Can you work these out from the model? Positions are in its coordinate system, mm. Face numbers are marked on the shaded views. A direction names the side the tool comes from. Give positions to 0.01 mm unless a question says otherwise; leave off trailing zeros. Loops run counter-clockwise (first coordinate to the right, second up) from the corner with the lowest first, then second, coordinate; pieces in that order, holes last. Notation, with made-up numbers: (68.25, 10.5) -> (84.25, 10.5) arc R27 cw to (84.25, 34.5) -> close; hole circle Ø8 at (7, 52.25). An arc over 180 degrees is marked (long way). Use CSV: the item, a comma, the result in double quotes.
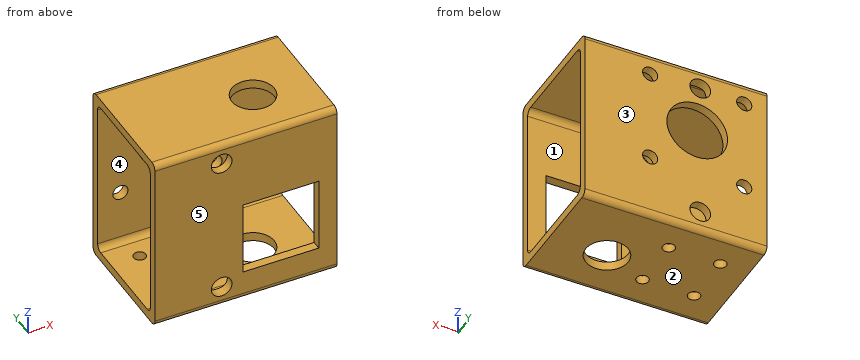
from build123d import *

# Parameters (mm, degrees)
EXTRUDE_1_DEPTH     = 60
CUT_EXTRUDE_1_REACH = 42
SKETCH_2_R          = 2.5
SKETCH_2_R_2        = 10
SKETCH_3_R          = 7
CUT_EXTRUDE_2_DEPTH = 61
HOLE_WIZARD_M8_1_D  = 6.8
CUT_EXTRUDE_3_REACH = 62
SKETCH_6_R          = 2
CUT_EXTRUDE_4_REACH = 42
SKETCH_7_W          = 25
SKETCH_7_H          = 25


with BuildPart() as part:
    # 草图1 → 凸台-拉伸1 (new body)
    with BuildSketch(Plane(origin=(0, 0, 0), x_dir=(0, 0, -1), z_dir=(1, 0, 0))):
        with BuildLine():
            Line((60, 2), (60, 38))
            ThreePointArc((60, 38), (59.414213562, 39.414213562), (58, 40))
            Line((58, 40), (2, 40))
            ThreePointArc((2, 40), (0.585786438, 39.414213562), (0, 38))
            Line((0, 38), (0, 2))
            ThreePointArc((0, 2), (0.585786438, 0.585786438), (2, 0))
            Line((2, 0), (58, 0))
            ThreePointArc((58, 0), (59.414213562, 0.585786438), (60, 2))
        make_face()
        with BuildLine():
            Line((3, 5), (3, 35))
            ThreePointArc((3, 35), (3.585786438, 36.414213562), (5, 37))
            Line((5, 37), (55, 37))
            ThreePointArc((55, 37), (56.414213562, 36.414213562), (57, 35))
            Line((57, 35), (57, 5))
            ThreePointArc((57, 5), (56.414213562, 3.585786438), (55, 3))
            Line((55, 3), (5, 3))
            ThreePointArc((5, 3), (3.585786438, 3.585786438), (3, 5))
        make_face(mode=Mode.SUBTRACT)
    extrude(amount=EXTRUDE_1_DEPTH)

    # 草图2 → 切除-拉伸1 (cut, up to next)
    with BuildSketch(Plane(origin=(0, 40, 0), x_dir=(1, 0, 0), z_dir=(0, 1, 0)), mode=Mode.PRIVATE) as cut_extrude_1_sk1:
        with Locations((7.5, 7.5)):
            Circle(SKETCH_2_R)
    cut_extrude_1_tool1 = extrude(cut_extrude_1_sk1.sketch, amount=-CUT_EXTRUDE_1_REACH, mode=Mode.PRIVATE) & part.part
    add(cut_extrude_1_tool1.solids().sort_by_distance((7.5, 40, -7.5))[0], mode=Mode.SUBTRACT)
    # 草图2 → 切除-拉伸1 (cut, up to next)
    with BuildSketch(Plane(origin=(0, 40, 0), x_dir=(1, 0, 0), z_dir=(0, 1, 0)), mode=Mode.PRIVATE) as cut_extrude_1_sk2:
        with Locations((38.5, 7.5)):
            Circle(SKETCH_2_R)
    cut_extrude_1_tool2 = extrude(cut_extrude_1_sk2.sketch, amount=-CUT_EXTRUDE_1_REACH, mode=Mode.PRIVATE) & part.part
    add(cut_extrude_1_tool2.solids().sort_by_distance((38.5, 40, -7.5))[0], mode=Mode.SUBTRACT)
    # 草图2 → 切除-拉伸1 (cut, up to next)
    with BuildSketch(Plane(origin=(0, 40, 0), x_dir=(1, 0, 0), z_dir=(0, 1, 0)), mode=Mode.PRIVATE) as cut_extrude_1_sk3:
        with Locations((38.5, 38.5)):
            Circle(SKETCH_2_R)
    cut_extrude_1_tool3 = extrude(cut_extrude_1_sk3.sketch, amount=-CUT_EXTRUDE_1_REACH, mode=Mode.PRIVATE) & part.part
    add(cut_extrude_1_tool3.solids().sort_by_distance((38.5, 40, -38.5))[0], mode=Mode.SUBTRACT)
    # 草图2 → 切除-拉伸1 (cut, up to next)
    with BuildSketch(Plane(origin=(0, 40, 0), x_dir=(1, 0, 0), z_dir=(0, 1, 0)), mode=Mode.PRIVATE) as cut_extrude_1_sk4:
        with Locations((7.5, 38.5)):
            Circle(SKETCH_2_R)
    cut_extrude_1_tool4 = extrude(cut_extrude_1_sk4.sketch, amount=-CUT_EXTRUDE_1_REACH, mode=Mode.PRIVATE) & part.part
    add(cut_extrude_1_tool4.solids().sort_by_distance((7.5, 40, -38.5))[0], mode=Mode.SUBTRACT)
    # 草图2 → 切除-拉伸1 (cut, up to next)
    with BuildSketch(Plane(origin=(0, 40, 0), x_dir=(1, 0, 0), z_dir=(0, 1, 0)), mode=Mode.PRIVATE) as cut_extrude_1_sk5:
        with Locations((23, 23)):
            Circle(SKETCH_2_R_2)
    cut_extrude_1_tool5 = extrude(cut_extrude_1_sk5.sketch, amount=-CUT_EXTRUDE_1_REACH, mode=Mode.PRIVATE) & part.part
    add(cut_extrude_1_tool5.solids().sort_by_distance((23, 40, -23))[0], mode=Mode.SUBTRACT)

    # 草图3 → 切除-拉伸2 (cut, through all)
    with BuildSketch(Plane.XY):
        with Locations((41, 17)):
            Circle(SKETCH_3_R)
    extrude(amount=-CUT_EXTRUDE_2_DEPTH, mode=Mode.SUBTRACT)

    # M8 螺纹孔1 (through all)
    with Locations(Plane(origin=(0, 40, 0), x_dir=(1, 0, 0), z_dir=(0, 1, 0))):
        with Locations((22, 53), (22, 7)):
            Hole(HOLE_WIZARD_M8_1_D / 2)

    # 草图6 → 切除-拉伸3 (cut, up to next)
    with BuildSketch(Plane(origin=(0, 0, -60), x_dir=(-1, 0, 0), z_dir=(0, 0, -1)), mode=Mode.PRIVATE) as cut_extrude_3_sk1:
        with Locations((-9.514718626, 11.514718626)):
            Circle(SKETCH_6_R)
    cut_extrude_3_tool1 = extrude(cut_extrude_3_sk1.sketch, amount=-CUT_EXTRUDE_3_REACH, mode=Mode.PRIVATE) & part.part
    add(cut_extrude_3_tool1.solids().sort_by_distance((9.514719, 11.514719, -60))[0], mode=Mode.SUBTRACT)
    # 草图6 → 切除-拉伸3 (cut, up to next)
    with BuildSketch(Plane(origin=(0, 0, -60), x_dir=(-1, 0, 0), z_dir=(0, 0, -1)), mode=Mode.PRIVATE) as cut_extrude_3_sk2:
        with Locations((-26.485281374, 11.514718626)):
            Circle(SKETCH_6_R)
    cut_extrude_3_tool2 = extrude(cut_extrude_3_sk2.sketch, amount=-CUT_EXTRUDE_3_REACH, mode=Mode.PRIVATE) & part.part
    add(cut_extrude_3_tool2.solids().sort_by_distance((26.485281, 11.514719, -60))[0], mode=Mode.SUBTRACT)
    # 草图6 → 切除-拉伸3 (cut, up to next)
    with BuildSketch(Plane(origin=(0, 0, -60), x_dir=(-1, 0, 0), z_dir=(0, 0, -1)), mode=Mode.PRIVATE) as cut_extrude_3_sk3:
        with Locations((-26.485281374, 28.485281374)):
            Circle(SKETCH_6_R)
    cut_extrude_3_tool3 = extrude(cut_extrude_3_sk3.sketch, amount=-CUT_EXTRUDE_3_REACH, mode=Mode.PRIVATE) & part.part
    add(cut_extrude_3_tool3.solids().sort_by_distance((26.485281, 28.485281, -60))[0], mode=Mode.SUBTRACT)
    # 草图6 → 切除-拉伸3 (cut, up to next)
    with BuildSketch(Plane(origin=(0, 0, -60), x_dir=(-1, 0, 0), z_dir=(0, 0, -1)), mode=Mode.PRIVATE) as cut_extrude_3_sk4:
        with Locations((-9.514718626, 28.485281374)):
            Circle(SKETCH_6_R)
    cut_extrude_3_tool4 = extrude(cut_extrude_3_sk4.sketch, amount=-CUT_EXTRUDE_3_REACH, mode=Mode.PRIVATE) & part.part
    add(cut_extrude_3_tool4.solids().sort_by_distance((9.514719, 28.485281, -60))[0], mode=Mode.SUBTRACT)

    # 草图7 → 切除-拉伸4 (cut, up to next)
    with BuildSketch(Plane.XZ, mode=Mode.PRIVATE) as cut_extrude_4_sk1:
        with Locations((41.5, -37.5)):
            Rectangle(SKETCH_7_W, SKETCH_7_H)
    cut_extrude_4_tool1 = extrude(cut_extrude_4_sk1.sketch, amount=-CUT_EXTRUDE_4_REACH, mode=Mode.PRIVATE) & part.part
    add(cut_extrude_4_tool1.solids().sort_by_distance((41.5, 0, -37.5))[0], mode=Mode.SUBTRACT)


solid = part.part
(1) Which directions (+Z, -Z, +X, -X, +Y, -Y) give clear straight access to the entire face, cutting with the end or side of a thin tool? Please do the marked faces 4 and 5.
Answer sheet:
face 4,"+X, -X"
face 5,"+Z, -Z, +X, -X, -Y"
(2) Will these pins go through, and if not, where does the flat tip stop? pin 1 Ø4 at (x, z) = (47, -37) entering from -Y; pin 2 Ø4 at (x, z) = (7.5, -38.5) entering from +Y; pin 3 Ø3 at (x, y) = (26.49, 11.51) entering from -Z.
Answer sheet:
pin 1,"stops at y = 37"
pin 2,"stops at y = 3"
pin 3,"stops at z = -3"
(3) If I drill on L1, parallel to Z at x = 22, y = 2.05; L2, parallel to Y at x = 8, z = -46; L3, parallel to Z at x = 18, y = 21, over which ranges is the centre line in solid material (lowest first)? Write a range as from..to.
Answer sheet:
L1,"z = -60..-56.4, -49.6..-10.4, -3.6..0"
L2,"y = 0..3, 37..40"
L3,"z = -60..-57, -3..0"
(4) If we section it at C-C, the plane z = -23: Write out the boundary of the cut face in (x, y), then the cut area to 3 significant figures.
Answer sheet:
outline,"(0, 0) -> (60, 0) -> (60, 3) -> (0, 3) -> close; (0, 37) -> (13, 37) -> (13, 40) -> (0, 40) -> close; (33, 37) -> (60, 37) -> (60, 40) -> (33, 40) -> close"
area,"300 mm2"
(5) If we section it at D-D, the plane y = 32: Write out the boundary of the cut face in (x, z).
Answer sheet:
outline,"(0, -60) -> (60, -60) -> (60, -57) -> (0, -57) -> close; (0, -3) -> (60, -3) -> (60, 0) -> (0, 0) -> close"
(6) If we section it at A-A, the plane x = 6: Write out the boundary of the cut face in (y, z), then the cut area to 3 significant figures.
Answer sheet:
outline,"(0, -58) arc R2 ccw to (2, -60) -> (38, -60) arc R2 ccw to (40, -58) -> (40, -40.5) -> (37, -40.5) -> (37, -55) arc R2 cw to (35, -57) -> (5, -57) arc R2 cw to (3, -55) -> (3, -5) arc R2 cw to (5, -3) -> (35, -3) arc R2 cw to (37, -5) -> (37, -5.5) -> (40, -5.5) -> (40, -2) arc R2 ccw to (38, 0) -> (2, 0) arc R2 ccw to (0, -2) -> close; (37, -36.5) -> (40, -36.5) -> (40, -9.5) -> (37, -9.5) -> close"
area,"540 mm2"
(7) We'd pull the mould along Z, two halves only. Please class the marked faces 1, 2 and 3: released by +Z, released by -Z, zero draft, split by the parting line, or undercut.
Answer sheet:
face 1,"undercut"
face 2,"released by -Z"
face 3,"zero draft"
(8) If we section it at B-B, the plane y = 17: Write out the boundary of the cut face in (x, z), then the cut area to 3 significant figures.
Answer sheet:
outline,"(0, -60) -> (34, -60) -> (34, -57) -> (0, -57) -> close; (0, -3) -> (34, -3) -> (34, 0) -> (0, 0) -> close; (48, -60) -> (60, -60) -> (60, -57) -> (48, -57) -> close; (48, -3) -> (60, -3) -> (60, 0) -> (48, 0) -> close"
area,"276 mm2"
